Source: CAD feature listing. Evaluate the final solid. Frame: model axes, mm. A direction names the side the tool comes from. Round coordinates to 2 decimals unless told otherwise and drop trailing zeros. Loops run counter-clockwise (first coordinate to the right, second up) from the corner with the lowest first, then second, coordinate; pieces in that order, holes last. Notation, with made-up numbers: M 76.25,67 L 125.25,67 A15 ccw 125.25,88 Z; hole C -23.75,-17.75 d3. An arc over 180 degrees is marked long. Answer as a JSON object with one key per item and string values.
from build123d import *

# Parameters (mm, degrees)
F1_DEPTH = 19.05
F3_DEPTH = 25.4
F5_DEPTH = 19.051


with BuildPart() as f1:
    # F0 (on Top) → F1 (new body)
    with BuildSketch(Plane.XY):
        with BuildLine():
            Line((14.9550589674, 50.2520292753), (-54.5516210822, 50.2520292753))
            Line((-54.5516210822, 50.2520292753), (-54.5516210822, 38.1094498451))
            Line((-54.5516210822, 38.1094498451), (-5.7937513614, 38.1094498451))
            ThreePointArc((-5.7937513614, 38.1094498451), (-0.1681561255, 34.7048153982), (-0.5750318579, 28.1417894487))
            Line((-0.5750318579, 28.1417894487), (-17.6851839396, 3.4592392383))
            Line((-17.6851839396, 3.4592392383), (14.9550589674, 50.2520292753))
        make_face()
        with BuildLine():
            ThreePointArc((-48.2016210822, 75.7045095678), (-52.6917491428, 73.8446376283), (-54.5516210822, 69.3545095678))
            Line((-54.5516210822, 69.3545095678), (-54.5516210822, 50.2520292753))
            Line((-54.5516210822, 50.2520292753), (14.9550589674, 50.2520292753))
            Line((14.9550589674, 50.2520292753), (-17.6851839396, 3.4592392383))
            Line((-17.6851839396, 3.4592392383), (-55.3482900739, -50.8723355951))
            ThreePointArc((-55.3482900739, -50.8723355951), (-56.1901550656, -52.5947874076), (-56.4795705704, -54.4899959914))
            Line((-56.4795705704, -54.4899959914), (-56.4795705704, -66.3977798347))
            ThreePointArc((-56.4795705704, -66.3977798347), (-54.6196986309, -70.8879078953), (-50.1295705704, -72.7477798347))
            Line((-50.1295705704, -72.7477798347), (48.2686518641, -72.7477798347))
            ThreePointArc((48.2686518641, -72.7477798347), (52.1466655513, -71.4260508936), (54.4102909159, -68.0110900211))
            Line((54.4102909159, -68.0110900211), (54.4102909159, -46.6400994718))
            Line((54.4102909159, -46.6400994718), (-18.9196563035, -46.6400994718))
            Line((-18.9196563035, -46.6400994718), (52.4497096213, 55.9125908699))
            Line((52.4497096213, 55.9125908699), (52.4497096213, 69.3545095678))
            ThreePointArc((52.4497096213, 69.3545095678), (50.5898376818, 73.8446376283), (46.0997096213, 75.7045095678))
            Line((46.0997096213, 75.7045095678), (-48.2016210822, 75.7045095678))
        make_face()
        with BuildLine():
            Line((52.4497096213, 35.9703072308), (52.4497096213, 55.9125908699))
            Line((52.4497096213, 55.9125908699), (-18.9196563035, -46.6400994718))
            Line((-18.9196563035, -46.6400994718), (54.4102909159, -46.6400994718))
            Line((54.4102909159, -46.6400994718), (54.4102909159, -68.0110900211))
            ThreePointArc((54.4102909159, -68.0110900211), (54.5663462033, -67.2111346224), (54.6186518641, -66.3977798347))
            Line((54.6186518641, -66.3977798347), (54.6186518641, -43.6716623549))
            ThreePointArc((54.6186518641, -43.6716623549), (52.7587799247, -39.1815342944), (48.2686518641, -37.3216623549))
            Line((48.2686518641, -37.3216623549), (15.5238411508, -37.3216623549))
            ThreePointArc((15.5238411508, -37.3216623549), (9.9045362797, -33.929011297), (10.2897481379, -27.3762805487))
            Line((10.2897481379, -27.3762805487), (51.3338026341, 32.3749254245))
            ThreePointArc((51.3338026341, 32.3749254245), (52.1643196925, 34.0880201421), (52.4497096213, 35.9703072308))
        make_face()
    extrude(amount=F1_DEPTH)

    # F2 (on face) → F3 (cut)
    with BuildSketch(Plane.XY.offset(19.05)):
        with BuildLine():
            ThreePointArc((44.2737464547, 65.4060840012), (44.0664205154, 66.5345943774), (43.4715192615, 67.5157224079))
            ThreePointArc((43.4715192615, 67.5157224079), (38.1310723939, 64.2775736249), (44.2737464547, 65.4060840012))
        make_face()
        with BuildLine():
            ThreePointArc((-40.3262716085, -64.7502714978), (-44.2935384673, -61.6757084029), (-46.2808783641, -66.2846805972))
            ThreePointArc((-46.2808783641, -66.2846805972), (-42.7090047498, -67.8248345927), (-40.3262716085, -64.7502714978))
        make_face()
    extrude(amount=-F3_DEPTH, mode=Mode.SUBTRACT)

    # F4 (on face) → F5 (cut, through all)
    with BuildSketch(Plane.XY.offset(19.05)):
        Polygon((42.4659381227, 60.1279996336), (36.9925759733, 61.0919743776), (-41.0894751549, 61.0919743776), (-41.0894751549, 47.3553165793), (20.6049866974, 47.3553165793), (-36.7515794933, -57.4770644307), (-36.7515794933, -65.4298663139), (43.9813993871, -65.4298663139), (43.9813993871, -44.9453778565), (-6.8683284335, -44.9453778565), (42.4659381227, 45.2243964511), align=None)
    extrude(amount=-F5_DEPTH, mode=Mode.SUBTRACT)


solid = f1.part
Item 1: Access query for faces 5 (the flat face through (52.45, 52, 9)), 6 (the flat face through (54.619, -55, 9)), 7 (the flat face through (-31, 38.109, 9)), 8 (the flat face through (30.524, 2.081, 9.392)), 9 (the flat face through (19, -44.945, 10)). Directions: +Z, -Z, +X, -X, +Y, -Y. A direction counts if a zero-diameter tool reaches every point of the face in a straight line with its end or side. Return the directions, or none.
Answer sheet:
{"face 5": "+Z, -Z, +X, +Y", "face 6": "+Z, -Z, +X, +Y, -Y", "face 7": "+Z, -Z, -X", "face 8": "+Z, -Z, +X", "face 9": "+Z, -Z"}
Item 2: Section B-B on x = 14. Return the cut outline in (y, z).
Answer sheet:
{"outline": "M -72.75,0 L -65.43,0 L -65.43,19.05 L -72.75,19.05 Z; M -44.95,0 L -37.14,0 L -37.14,19.05 L -44.95,19.05 Z; M -21.97,0 L -6.8,0 L -6.8,19.05 L -21.97,19.05 Z; M 35.28,0 L 47.36,0 L 47.36,19.05 L 35.28,19.05 Z; M 61.09,0 L 75.7,0 L 75.7,19.05 L 61.09,19.05 Z"}
Item 3: Contact query for flat-ended pins moving along their axis: pin 1 Ø4 at (x, y) = (41.1, 65.41) entering from -Z; pin 2 Ø4 at (y, z) = (45, 14.5) entering from -X; pin 3 Ø6 at (x, y) = (-17, 6) entering from +Z; pin 4 Ø8 at (y, z) = (19, 9.5) entering from +X. Output: stop coordinate, or through.
Answer sheet:
{"pin 1": "passes through", "pin 2": "stops at x = -54.55", "pin 3": "stops at z = 19.05", "pin 4": "stops at x = 44.89"}
Item 4: Pull-direction query (X, two-part tool) for faces 1 (the flat face through (-1, 13, 0)), 2 (the cylindrical face through (52.808, -39.231, 9.392)), 3 (the flat face through (39.768, 60.603, 9.658)), 4 (the flat face through (-7.672, -4.327, 9.658)); classes: pulls with the +X half, pulls with the -X half, needs draft (parallel to the pull), parting line crosses it, or undercut.
Answer sheet:
{"face 1": "needs draft", "face 2": "pulls with the +X half", "face 3": "undercut", "face 4": "undercut"}
Item 5: Section C-C on x = -33.5. Return the cut outline in (y, z).
Answer sheet:
{"outline": "M -72.75,0 L -65.43,0 L -65.43,19.05 L -72.75,19.05 Z; M -51.53,0 L -19.35,0 L -19.35,19.05 L -51.53,19.05 Z; M 38.11,0 L 47.36,0 L 47.36,19.05 L 38.11,19.05 Z; M 61.09,0 L 75.7,0 L 75.7,19.05 L 61.09,19.05 Z"}
Item 6: Line query: probe 1 along Y at (x, z) = (27.5, 14.5); probe 2 along Y at (x, z) = (6, 17.25); probe 3 along X at (y, z) = (50, 4.5). Output: solid intervals per line, ascending. Write a range as from..to.
Answer sheet:
{"probe 1": "y = -72.75..-65.43, -44.95..-37.32, -2.32..17.87, 61.09..75.7", "probe 2": "y = -72.75..-65.43, -44.95..-21.43, 20.66..47.36, 61.09..75.7", "probe 3": "x = -54.55..-41.09, 42.47..52.45"}
Item 7: Section A-A on y = 5. Return the cut outline in (x, z).
Answer sheet:
{"outline": "M -16.62,0 L -2.57,0 L -2.57,19.05 L -16.62,19.05 Z; M 20.46,0 L 32.53,0 L 32.53,19.05 L 20.46,19.05 Z"}
Item 8: Section D-D on z = 8.5. Give the number of separate pieces and of enclosed holes in the cut face, then the cut area to 3 significant figures.
Answer sheet:
{"separate pieces": "1", "enclosed holes": "3", "area": "6,660 mm²"}
